```python
from build123d import *

# Parameters (mm, degrees)
SKETCH1_R           = 1.5
BOSS_EXTRUDE1_DEPTH = 12
SKETCH2_R           = 2.75
BOSS_EXTRUDE2_DEPTH = 3
FILLET1_R           = 0.2
FILLET2_R           = 0.1
FILLET3_R           = 0.1


with BuildPart() as part:
    # Sketch1 → Boss-Extrude1 (new body)
    with BuildSketch(Plane(origin=(0, 0, 0), x_dir=(1, 0, 0), z_dir=(0, 1, 0))):
        with Locations(Location((0, 0, 0), (0, 0, 270))):
            Circle(SKETCH1_R)
    extrude(amount=BOSS_EXTRUDE1_DEPTH)

    # Sketch2 → Boss-Extrude2 (add)
    with BuildSketch(Plane(origin=(0, 12, 0), x_dir=(1, 0, 0), z_dir=(0, 1, 0))):
        with Locations(Location((0, 0, 0), (0, 0, 270))):
            Circle(SKETCH2_R)
    extrude(amount=BOSS_EXTRUDE2_DEPTH)

    # Fillet1
    fillet1_edges = [part.edges().sort_by_distance(p)[0] for p in [
        (0, 12, -1.5),
    ]]
    fillet(fillet1_edges, radius=FILLET1_R)

    # Fillet2
    fillet2_edges = [part.edges().sort_by_distance(p)[0] for p in [
        (0, 15, -2.75),
    ]]
    fillet(fillet2_edges, radius=FILLET2_R)

    # Fillet3
    fillet3_edges = [part.edges().sort_by_distance(p)[0] for p in [
        (0, 12, -2.75),
    ]]
    fillet(fillet3_edges, radius=FILLET3_R)


solid = part.part
```
Can you work these out from the model? Positions are in its coordinate system, mm. A direction names the side the tool comes from. Coordinates: 2 decimals unless noted, no trailing zeros. Loops run counter-clockwise (first coordinate to the right, second up) from the corner with the lowest first, then second, coordinate; pieces in that order, holes last. Notation, with made-up numbers: (29, 35) - (52, 35) arc R33 cw to (52, 70) - close; hole circle Ø7 at (87.25, 69.5). An arc over 180 degrees is marked (long way). Use a Markdown table: item, result.
Item 1: I want a section at B-B on x = 0. Please give me the cut outline in (y, z).
Numbers:
| item | result |
|---|---|
| outline | (0, -1.5) - (11.8, -1.5) arc R0.2 cw to (12, -1.7) - (12, -2.65) arc R0.1 ccw to (12.1, -2.75) - (14.9, -2.75) arc R0.1 ccw to (15, -2.65) - (15, 2.65) arc R0.1 ccw to (14.9, 2.75) - (12.1, 2.75) arc R0.1 ccw to (12, 2.65) - (12, 1.7) arc R0.2 cw to (11.8, 1.5) - (0, 1.5) - close |
Item 2: I want a section at C-C on y = 13.5. Please give me the cut outline in (x, z), and give its area (3 significant figures).
Numbers:
| item | result |
|---|---|
| outline | circle Ø5.5 at (0, 0) |
| area | 23.8 mm2 |
Item 3: For faces 1 (the face through (-2.685, 13.48, -0.596)), 2 (the face through (0, 12, 2)), which set-ups out of +Z, -Z, +X, -X, +Y, -Y let a thin tool reach every point of the face, with its end or its side?
Numbers:
| item | result |
|---|---|
| face 1 | +Y, -Y |
| face 2 | -Y |
Item 4: If I drill on probe 1 along Y at (x, z) = (0.15, -2.3); probe 2 along X at (y, z) = (12.75, -0.7); probe 3 along X at (y, z) = (8.5, -1.05), over which ranges is the centre line in solid material (lowest first)? Write a range as from..to.
Numbers:
| item | result |
|---|---|
| probe 1 | y = 12..15 |
| probe 2 | x = -2.66..2.66 |
| probe 3 | x = -1.07..1.07 |
Item 5: I want a section at A-A on z = 0. Please give me the cut outline in (x, y), and give its area (3 significant figures).
Numbers:
| item | result |
|---|---|
| outline | (-2.75, 12.1) arc R0.1 ccw to (-2.65, 12) - (-1.7, 12) arc R0.2 cw to (-1.5, 11.8) - (-1.5, 0) - (1.5, 0) - (1.5, 11.8) arc R0.2 cw to (1.7, 12) - (2.65, 12) arc R0.1 ccw to (2.75, 12.1) - (2.75, 14.9) arc R0.1 ccw to (2.65, 15) - (-2.65, 15) arc R0.1 ccw to (-2.75, 14.9) - close |
| area | 52.5 mm2 |
Item 6: I want a section at D-D on y = 5. Please give me the cut outline in (x, z).
Numbers:
| item | result |
|---|---|
| outline | circle Ø3 at (0, 0) |
Item 7: Will these pins go through, and if not, where does the flat tip stop? pin 1 (3 mm diameter, centred on x = 1, z = -1.5, fed in from -Y); pin 2 (1.5 mm diameter, centred on x = 0, y = 8.5, fed in from -Z).
Numbers:
| item | result |
|---|---|
| pin 1 | stops at y = 0 |
| pin 2 | stops at z = -1.5 |
